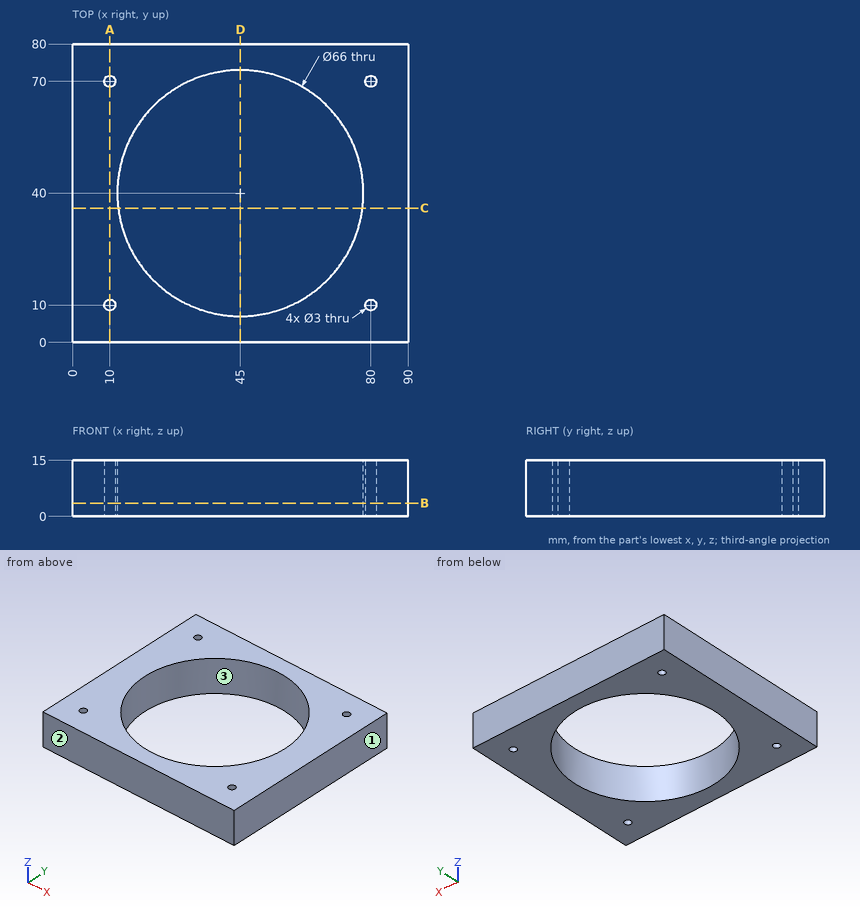
Geometry: see drawing. Coordinates: mm, zero at the bounding-box minimum. Round coordinates to 2 decimals unless told otherwise and drop trailing zeros. Loops run counter-clockwise (first coordinate to the right, second up) from the corner with the lowest first, then second, coordinate; pieces in that order, holes last. Notation, with made-up numbers: (24, 77.5) -> (58, 77.5) arc R23 cw to (58, 95.5) -> close; hole circle Ø9 at (-18, -28.75). An arc over 180 degrees is marked (long way). Write each question's results on one line, items separated by ' | '.
1. Ray query, line 1 (Y direction, x = 80, z = 6.5); line 2 (X direction, y = 10, z = 5); line 3 (Y direction, x = 23.5, z = 6). Return the intervals inside material, ascending. Write a range as from..to.
Geometry results:
line 1: 0..8.5, 11.5..68.5, 71.5..80 | line 2: 0..8.5, 11.5..31.25, 58.75..78.5, 81.5..90 | line 3: 0..14.97, 65.03..80
2. Section D-D (x = 45). Return loops of the section in (y, z).
Geometry results:
outline: (0, 0) -> (7, 0) -> (7, 15) -> (0, 15) -> close; (73, 0) -> (80, 0) -> (80, 15) -> (73, 15) -> close
3. Mould query, pull axis Y, two halves, no side actions, for the marked faces 1, 2 and 3. Classes: +Y half, -Y half, draft (parallel to the pull), parting line (faces both ways), or undercut.
Geometry results:
face 1: draft | face 2: -Y half | face 3: undercut
4. Section C-C (y = 36). Return loops of the section in (x, z), and give its area (3 significant figures).
Geometry results:
outline: (0, 0) -> (12.24, 0) -> (12.24, 15) -> (0, 15) -> close; (77.76, 0) -> (90, 0) -> (90, 15) -> (77.76, 15) -> close | area: 367 mm2
5. First-contact query: P1, Ø1.8, axis at x = 10, y = 70, coming from the -Z side. Flat tip, straight axial feed; report the tip coordinate or a pass-through.
Geometry results:
P1: through
6. Section A-A (x = 10). Return loops of the section in (y, z), and give its area (3 significant figures).
Geometry results:
outline: (0, 0) -> (8.5, 0) -> (8.5, 15) -> (0, 15) -> close; (11.5, 0) -> (68.5, 0) -> (68.5, 15) -> (11.5, 15) -> close; (71.5, 0) -> (80, 0) -> (80, 15) -> (71.5, 15) -> close | area: 1,110 mm2
7. Section B-B (z = 3.5). Return loops of the section in (x, y), and give its area (3 significant figures).
Geometry results:
outline: (0, 0) -> (90, 0) -> (90, 80) -> (0, 80) -> close; hole circle Ø3 at (10, 10); hole circle Ø3 at (10, 70); hole circle Ø66 at (45, 40); hole circle Ø3 at (80, 10); hole circle Ø3 at (80, 70) | area: 3,750 mm2
